Here's how the part is built. I have some questions about the finished solid (model axes, mm). Face numbers are marked on the shaded views. A direction names the side the tool comes from. Coordinates: 2 decimals unless noted, no trailing zeros. Write each loop counter-clockwise with the first axis right and the second up, starting at its lowest first coordinate (ties: lowest second). Pieces come first, ordered by that corner, then holes.
(1) Imagine slicing it at C-C, the plane z = 6.75. List the corners of the cut face in (x, y) for me, plus the area to 3 significant figures.
(2) Which directions (+Z, -Z, +X, -X, +Y, -Y) give clear straight access to the entire face, cutting with the end or side of a thin tool? Please do the marked faces 1 and 2.
(3) For pin 1 Ø1 at (x, y) = (-40.5, -30.5) entering from +Z; pin 2 Ø0.6 at (x, z) = (-36.5, 0.5) entering from -Y; pin 3 Ø1 at (x, z) = (-43.5, 2) entering from +Y; pin 4 Ø1.3 at (x, y) = (-36, -19.5) entering from -Z, each with a flat end and sliding along its axis, tell me the tip position at first contact or that it passes through.
(4) Please list where these lines run through material, in increasing order: probe 1 along Z at (x, y) = (-31, -27.25); probe 2 along Z at (x, y) = (-41.25, -19.5); probe 3 along Y at (x, z) = (-33.5, 2).
(5) Imagine slicing it at A-A, the plane x = -30.75. List the corners of the cut face in (y, z) for me.
(6) Imagine slicing it at D-D, the plane y = -23.5. List the corners of the cut face in (x, z) for me.
(7) Imagine slicing it at B-B, the plane y = -20.25. List the corners of the cut face in (x, z) for me.
```python
from build123d import *

# Parameters (mm, degrees)
F0_R      = 4.325
F1_DEPTH  = 3
F0_R_2    = 5
F1_FACE_R = 4.325
F2_DEPTH  = 0.7
F0_R_3    = 13.1400703873
F0_R_4    = 6.4331806046
F0_R_5    = 4.3173351149
F3_DEPTH  = 8
F4_DEPTH  = 3
F7_W      = 1.5792734921
F7_H      = 3.3408720046
F8_DEPTH  = 0.5


with BuildPart() as f1:
    # F0 (on Top) → F1 (new body)
    with BuildSketch(Plane.XY):
        Circle(F0_R)
    extrude(amount=-F1_DEPTH)

    # F0 (on Top) + F1_face (on face) → F2 (join)
    with BuildSketch(Plane.XY):
        Circle(F0_R_2)
        Circle(F0_R, mode=Mode.SUBTRACT)
    with BuildSketch(Plane.XY):
        Circle(F1_FACE_R)
    extrude(amount=F2_DEPTH)


with BuildPart() as f2:
    # F0 (on Top) → F2, piece 2 (new body)
    with BuildSketch(Plane.XY):
        with Locations((-35.7068367302, -21.6784439981)):
            Circle(F0_R_3)
        with Locations((-35.7068367302, -21.6784439981)):
            Circle(F0_R_4, mode=Mode.SUBTRACT)
    extrude(amount=F2_DEPTH)


with BuildPart() as f3:
    # F0 (on Top) → F3 (new body)
    with BuildSketch(Plane.XY):
        with Locations((-35.7068367302, -21.6784439981)):
            Circle(F0_R_5)
    extrude(amount=F3_DEPTH)


with BuildPart() as f4:
    # F0 (on Top) → F4 (new body)
    with BuildSketch(Plane.XY):
        with Locations((-35.7068367302, -21.6784439981)):
            Circle(F0_R_4)
        with Locations((-35.7068367302, -21.6784439981)):
            Circle(F0_R_5, mode=Mode.SUBTRACT)
    extrude(amount=F4_DEPTH)


with BuildPart() as f2_1:
    add(f2.part)

    # F6: union F3, F4
    add(f3.part)
    add(f4.part)

    # F7 (on face) → F8 (cut)
    with BuildSketch(Plane(origin=(0, 0, 0), x_dir=(1, 0, 0), z_dir=(0, 0, -1))):
        with Locations((-36.0395330936, 20.4883767292)):
            Rectangle(F7_W, F7_H)
    extrude(amount=-F8_DEPTH, mode=Mode.SUBTRACT)


solid = f2_1.part
```
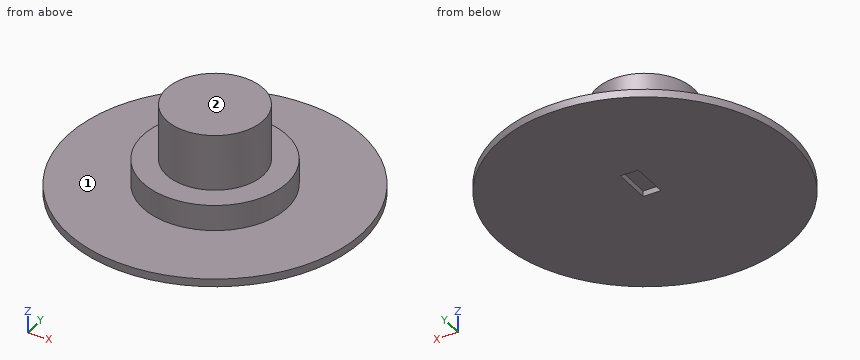
Recorded:
1. outline: circle Ø8.63 at (-35.71, -21.68)
1. area: 58.6 mm2
2. face 1: +Z
2. face 2: +Z, +X, -X, +Y, -Y
3. pin 1: stops at z = 0.7
3. pin 2: stops at y = -34.81
3. pin 3: passes through
3. pin 4: stops at z = 0.5
4. probe 1: z = 0 to 0.7
4. probe 2: z = 0 to 3
4. probe 3: y = -27.72 to -15.64
5. outline: (-33.85, 0) - (-9.51, 0) - (-9.51, 0.7) - (-17.58, 0.7) - (-17.58, 3) - (-25.78, 3) - (-25.78, 0.7) - (-33.85, 0.7) - close
6. outline: (-48.72, 0) - (-22.69, 0) - (-22.69, 0.7) - (-29.54, 0.7) - (-29.54, 3) - (-31.79, 3) - (-31.79, 8) - (-39.62, 8) - (-39.62, 3) - (-41.88, 3) - (-41.88, 0.7) - (-48.72, 0.7) - close
7. outline: (-48.77, 0) - (-36.83, 0) - (-36.83, 0.5) - (-35.25, 0.5) - (-35.25, 0) - (-22.64, 0) - (-22.64, 0.7) - (-29.43, 0.7) - (-29.43, 3) - (-31.63, 3) - (-31.63, 8) - (-39.78, 8) - (-39.78, 3) - (-41.98, 3) - (-41.98, 0.7) - (-48.77, 0.7) - close
